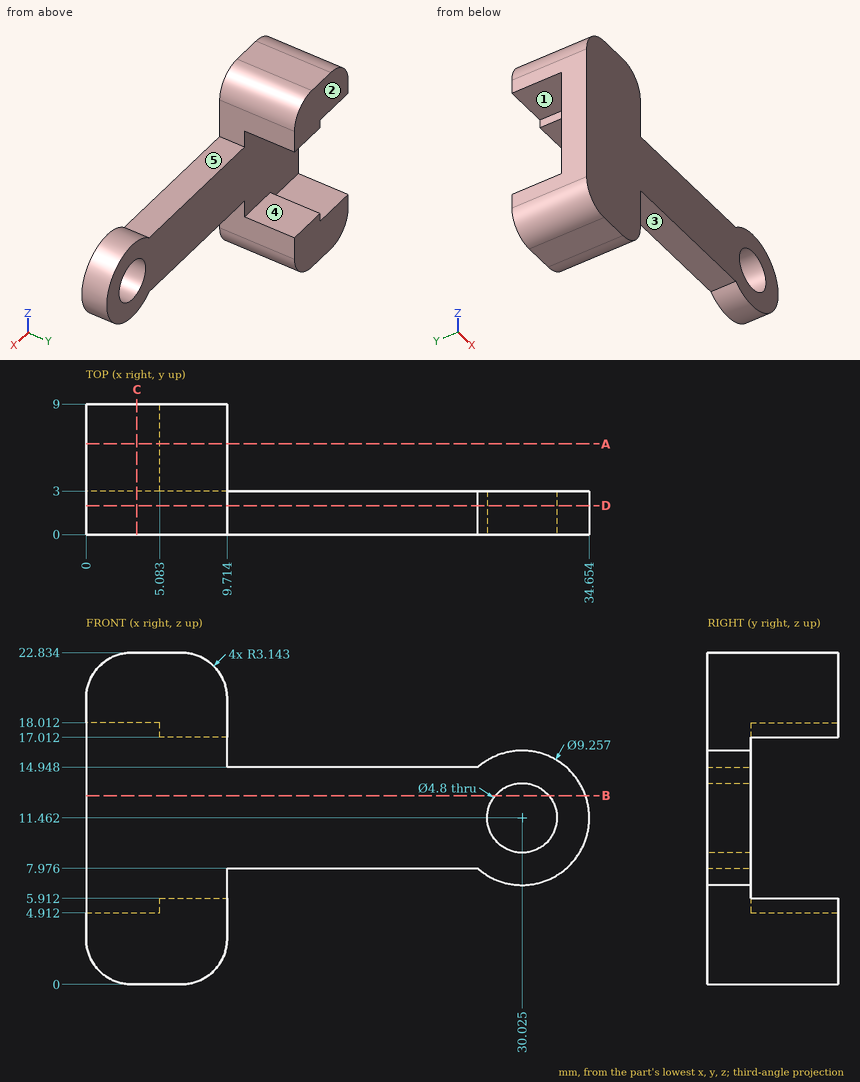
Answer from the drawing. Dimensions are ordinates in mm from the lowest x, y and z of the part. A direction names the side the tool comes from. Coordinates: 2 decimals unless noted, no trailing zeros. Loops run counter-clockwise (first coordinate to the right, second up) from the corner with the lowest first, then second, coordinate; pieces in that order, holes last.
1) Flat-ended cylindrical pins translate along their axes: pin 1 (0.8 mm diameter, centred on y = 6.5, z = 5.5, fed in from -X); pin 2 (2.5 mm diameter, centred on x = 15.5, y = 1.5, fed in from -Z); pin 3 (4 mm diameter, centred on y = 6.5, z = 5.5, fed in from +X); pin 4 (2 mm diameter, centred on y = 5.5, z = 7.5, fed in from +X). Find the tip coordinate at first contact, or state that the pin passes through.
Results:
pin 1: stops at x = 5.08
pin 2: stops at z = 7.98
pin 3: stops at x = 9.71
pin 4: passes through
2) Consider probe 1 along Y at (x, z) = (21, 13); probe 2 along Z at (x, y) = (17.5, 2.25); probe 3 along Z at (x, y) = (8, 4) (1 decimal). Determine where each line is inside the solid, lowest interval first.
Results:
probe 1: y = 0 to 3
probe 2: z = 7.98 to 14.95
probe 3: z = 0.3 to 5.9, 17 to 22.5
3) Section B-B (z = 13) is taken. Give the vertices of the cut face in (x, y).
Results:
outline: (0, 0) - (28.18, 0) - (28.18, 3) - (0, 3) - close; (31.87, 0) - (34.39, 0) - (34.39, 3) - (31.87, 3) - close
4) Section C-C (x = 3.5) is taken. Give the vertices of the cut face in (y, z).
Results:
outline: (0, 0) - (9, 0) - (9, 4.91) - (3, 4.91) - (3, 18.01) - (9, 18.01) - (9, 22.83) - (0, 22.83) - close
5) Section D-D (y = 2) is taken. Give the vertices of the cut face in (x, z) (1 decimal).
Results:
outline: (0, 3.1) arc R3.1 ccw to (3.1, 0) - (6.6, 0) arc R3.1 ccw to (9.7, 3.1) - (9.7, 8) - (27, 8) arc R4.6 ccw (long way) to (27, 14.9) - (9.7, 14.9) - (9.7, 19.7) arc R3.1 ccw to (6.6, 22.8) - (3.1, 22.8) arc R3.1 ccw to (0, 19.7) - close; hole circle Ø4.8 at (30, 11.5)
6) For the marked faces 1, 2, 3, 4 and 5, determine the directions among +Z, -Z, +X, -X, +Y, -Y from which every point of the face is accessible in a straight line to the end or side of a thin tool.
Results:
face 1: -X, +Y
face 2: +Z, -Z, +X, -X, +Y
face 3: -Z, +Y, -Y
face 4: +X, -X, +Y
face 5: +Z, +Y, -Y
7) Section A-A (y = 6.25) is taken. Give the vertices of the cut face in (x, z) (1 decimal).
Results:
outline: (0, 3.1) arc R3.1 ccw to (3.1, 0) - (6.6, 0) arc R3.1 ccw to (9.7, 3.1) - (9.7, 5.9) - (5.1, 5.9) - (5.1, 4.9) - (0, 4.9) - close; (0, 18) - (5.1, 18) - (5.1, 17) - (9.7, 17) - (9.7, 19.7) arc R3.1 ccw to (6.6, 22.8) - (3.1, 22.8) arc R3.1 ccw to (0, 19.7) - close
